For this review, take the finished solid that the model builds, in its own axes (mm). Give positions to 0.01 mm unless a question says otherwise; leave off trailing zeros. Loops run counter-clockwise (first coordinate to the right, second up) from the corner with the lowest first, then second, coordinate; pieces in that order, holes last.
Autodesk Inventor part; units mm, degrees
ref_plane "YZ Plane" through (0, 0, 0) normal (1, 0, 0) x (0, 1, 0)
ref_plane "XZ Plane" through (0, 0, 0) normal (0, 1, 0) x (-1, 0, 0)
ref_plane "XY Plane" through (0, 0, 0) normal (0, 0, 1) x (1, 0, 0)
sketch "Sketch1" plane through (0, 0, 0) normal (0, 0, 1) x (1, 0, 0)
  circle A0 centre (0, 0) radius 17.4625
  circle A1 centre (0, 0) radius 18.2245
  dimension "d0" = 34.925
  dimension "d1" = 36.449
extrude "Extrusion1" add sketch "Sketch1" along normal blind 19.05
sketch "Sketch2" plane through (0, 0, 19.05) normal (0, 0, 1) x (1, 0, 0)
  circle A0 centre (0, 0) radius 18.2245
  line L0 (0, 18.2245) -> (0, 17.4625)
  circle A1 centre (0, 0) radius 17.4625
  line L1 (0.7937, 18.2072) -> (0.7937, 17.4445)
  dimension "d4" = 0.7937
extrude "Extrusion2" cut sketch "Sketch2" against normal blind 19.05 contours L1 A1 L0 A0 picked at (0.7055, 17.702)
properties part number "Buffer" material "PBT Plastic"
Item 1: Take a section at B-B on x = -5. Give the boundary of the cut face in (y, z).
Answer:
outline: (-17.53, 0) - (-16.73, 0) - (-16.73, 19.05) - (-17.53, 19.05) - close; (16.73, 0) - (17.53, 0) - (17.53, 19.05) - (16.73, 19.05) - close
Item 2: For L1, parallel to X at y = 0, z = 11; L2, parallel to X at y = -8, z = 1.25; L3, parallel to Y at x = -9, z = 18.25, list the stretches that pass through material, from the lowest coordinate up.
Answer:
L1: x = -18.22 to -17.46, 17.46 to 18.22
L2: x = -16.37 to -15.52, 15.52 to 16.37
L3: y = -15.85 to -14.96, 14.96 to 15.85
Item 3: Take a section at C-C on z = 8. Give the boundary of the cut face in (x, y) (1 decimal), and give its area (3 significant figures).
Answer:
outline: (0, 17.5) - (0, 18.2) arc R18.2 ccw (long way) to (0.8, 18.2) - (0.8, 17.4) arc R17.5 cw (long way) to start
area: 84.8 mm2
Item 4: Take a section at A-A on y = -11. Give the boundary of the cut face in (x, z).
Answer:
outline: (-14.53, 0) - (-13.56, 0) - (-13.56, 19.05) - (-14.53, 19.05) - close; (13.56, 0) - (14.53, 0) - (14.53, 19.05) - (13.56, 19.05) - close
Item 5: Clearance check with flat-ended pins moving along their axes: pin 1 Ø8 at (x, z) = (7, 13.5) entering from +Y; pin 2 Ø5 at (x, z) = (13, 15.5) entering from +Y; pin 3 Ø5 at (x, z) = (3.5, 16) entering from +Y; pin 4 Ø6 at (x, y) = (13.5, -2.5) entering from +Z. State where each tip first meets the part, or that it passes through.
Answer:
pin 1: stops at y = 17.98
pin 2: stops at y = 14.9
pin 3: stops at y = 18.2
pin 4: passes through
